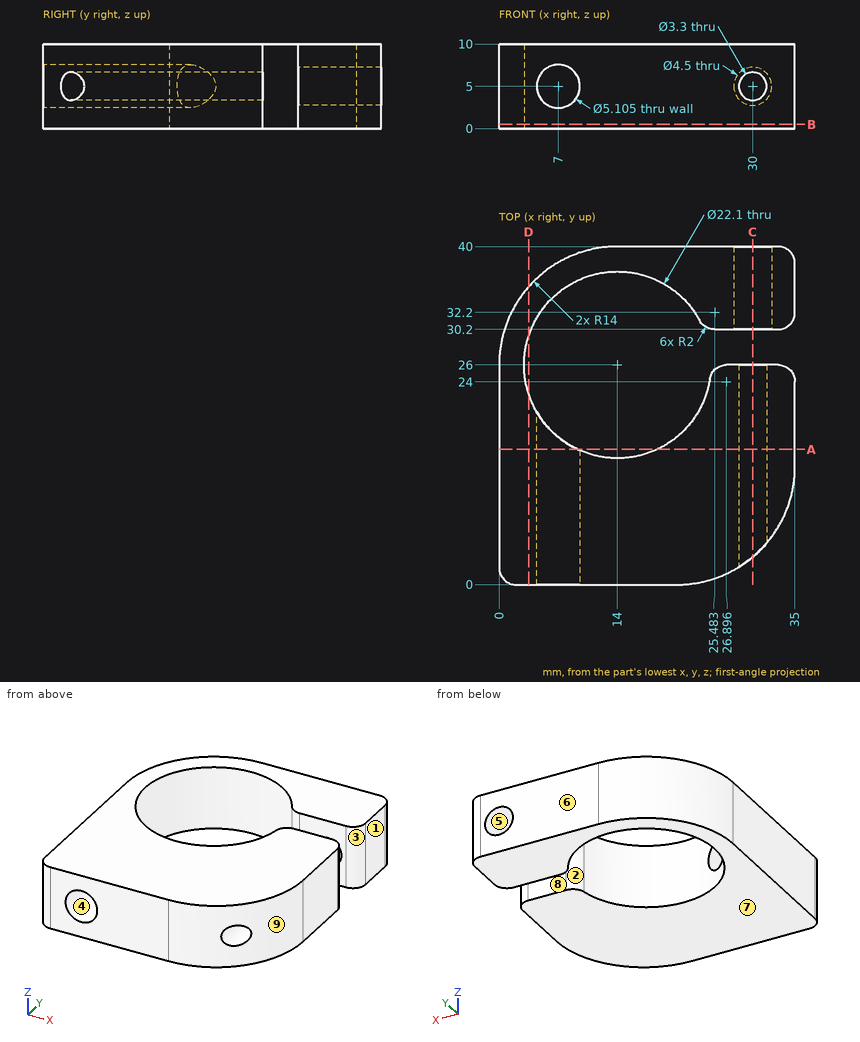
Check sheet for the drawn part. Datum: minimum x, y, z corner. Units: mm. A direction names the side the tool comes from. Give positions to 0.01 mm unless a question says otherwise; leave off trailing zeros. Loops run counter-clockwise (first coordinate to the right, second up) from the corner with the lowest first, then second, coordinate; pieces in that order, holes last.
1) Depth check by flat-ended pin: pin 1 Ø4 at (x, z) = (7, 5) entering from -Y; pin 2 Ø1.8 at (x, z) = (31, 6.5) entering from +Y; pin 3 Ø6 at (x, z) = (30.5, 4.5) entering from -Y; pin 4 Ø3 at (x, z) = (30, 5) entering from -Y. Enter the tip coordinate at first touch or a pass-through.
2) Sectioned sample at D-D, the plane x = 3.5. Enter the section's corners in (y, z), then the cut area to 3 significant figures.
3) Sectioned sample at A-A, the plane y = 16. Count the separate pieces of the cut face and the enclosed holes in it, then the cut area to 3 significant figures.
4) Set-up check for the marked faces 1, 2, 3, 4 and 5: record each of +Z, -Z, +X, -X, +Y, -Y from which the full face is reachable in a straight line by a thin tool's end or side.
5) Draft check along Y on the marked faces 6, 7, 8 and 9. Enter one of: pulls with the +Y half, pulls with the -Y half, needs draft (parallel to the pull), parting line crosses it, or undercut.
6) Sectioned sample at C-C, the plane x = 30. Enter the section's corners in (y, z).
7) Thickness scan on line 1 along Z through (x, y) = (30, 13); line 2 along Z through (x, y) = (30, 32.5); line 3 along Y through (x, z) = (14, 7). Record the ranges inside material, lowest first.
8) Sectioned sample at B-B, the plane z = 0.5. Enter the section's corners in (x, y).
Answers:
1. pin 1: stops at y = 32.41
1. pin 2: stops at y = 40
1. pin 3: stops at y = 1.6
1. pin 4: passes through
2. outline: (0, 0) - (22.56, 0) - (22.56, 10) - (0, 10) - close; (29.44, 0) - (35.26, 0) - (35.26, 10) - (29.44, 10) - close
2. area: 284 mm2
3. separate pieces: 2
3. enclosed holes: 1
3. area: 227 mm2
4. face 1: +Z, -Z, +X, +Y, -Y
4. face 2: +Z, -Z
4. face 3: +Z, -Z, +X
4. face 4: -Y
4. face 5: +Y
5. face 6: pulls with the +Y half
5. face 7: needs draft
5. face 8: undercut
5. face 9: pulls with the -Y half
6. outline: (3.28, 0) - (26, 0) - (26, 3.35) - (3.28, 3.35) - close; (3.28, 6.65) - (26, 6.65) - (26, 10) - (3.28, 10) - close; (30.2, 0) - (40, 0) - (40, 2.75) - (30.2, 2.75) - close; (30.2, 7.25) - (40, 7.25) - (40, 10) - (30.2, 10) - close
7. line 1: z = 0 to 3.35, 6.65 to 10
7. line 2: z = 0 to 2.75, 7.25 to 10
7. line 3: y = 0 to 14.95, 37.05 to 40
8. outline: (0, 2) arc R2 ccw to (2, 0) - (21, 0) arc R14 ccw to (35, 14) - (35, 24) arc R2 ccw to (33, 26) - (26.9, 26) arc R2 ccw to (24.92, 24.31) arc R11.05 cw (long way) to (23.72, 31.25) arc R2 ccw to (25.48, 30.2) - (33, 30.2) arc R2 ccw to (35, 32.2) - (35, 38) arc R2 ccw to (33, 40) - (14, 40) arc R14 ccw to (0, 26) - close
